Could you check a few things on this model? Use its own coordinates, in mm. A direction names the side the tool comes from. Give positions to 0.01 mm unless a question says otherwise; leave off trailing zeros. Loops run counter-clockwise (first coordinate to the right, second up) from the corner with the lowest first, then second, coordinate; pieces in that order, holes last. Notation, with made-up numbers: (-12.5, -39.5) - (5.5, -39.5) arc R20 ccw to (5.5, -35.5) - close; hole circle Ø10 at (9, 84). An arc over 180 degrees is marked (long way). One line per item, written item: value. Start each with the question number.
Q1. I want a section at B-B (y = -103.5). Please give me the cut outline in (x, z) (3 decimals).
Q2. I want a section at C-C (x = 100). Please give me the cut outline in (y, z) (3 decimals).
Q3. I'm going to push flat-ended pins straight in: P1, Ø6, axis at x = 45, z = 34.5, coming from the +Y side; P2, Ø18.5, axis at y = -9, z = 2, coming from the +X side; P3, Ø23, axis at x = 70.5, y = 7, coming from the -Z side (3 decimals). Where does each tip first touch, or does it pass through?
Q4. I want a section at A-A (z = 76.5). Please give me the cut outline in (x, y), then the cut area to 3 significant figures.
Q5. If I drill on line 1 (Z direction, x = 33.5, y = 68) (3 decimals); line 2 (Y direction, x = 41, z = 34.5); line 3 (X direction, y = -1.5, z = 75), over which ranges is the centre line in solid material (lowest first)? Write a range as from..to.
Q6. For faces 1 (the face through (88, 0, 15.875)), 2 (the face through (110.693, -9.728, 67.386)), 3 (the face through (33.269, 16.547, 50.986)), 4 (the face through (61, -2, 61.925)), 5 (the face through (23.73, -17, 18)), which set-ups out of +Z, -Z, +X, -X, +Y, -Y let a thin tool reach every point of the face, with its end or its side?
```python
from build123d import *

# Parameters (mm, degrees)
F1_DEPTH = 127
F0_W     = 25.4
F0_H     = 19.05
F2_DEPTH = 25.4
F3_DEPTH = 7.9375
F5_R     = 12.7


with BuildPart() as f1:
    # F0 (on Front) → F1 (new body, symmetric)
    with BuildSketch(Plane.XZ):
        Polygon((23.7298189036, 9.525), (-39.7701810964, 9.525), (-39.7701810964, -9.525), (42.7798189036, -9.525), (42.7798189036, 9.525), align=None)
    extrude(amount=F1_DEPTH, both=True)

    # F0 (on Front) → F2 (join, symmetric)
    with BuildSketch(Plane.XZ):
        with Locations((74.5298189036, 52.4002)):
            Rectangle(F0_W, F0_H)
        with BuildLine():
            Line((23.7298189036, 27.0002), (23.7298189036, 9.525))
            Line((23.7298189036, 9.525), (42.7798189036, 9.525))
            Line((42.7798189036, 9.525), (42.7798189036, 27.0002))
            ThreePointArc((42.7798189036, 27.0002), (47.4294987522, 38.2255201513), (58.6548189036, 42.8752))
            Line((58.6548189036, 42.8752), (61.8298189036, 42.8752))
            Line((61.8298189036, 42.8752), (61.8298189036, 61.9252))
            Line((61.8298189036, 61.9252), (58.6548189036, 61.9252))
            add(Edge.make_bspline(
                [(55.9463563883, 61.8200198703), (56.8425826502, 61.8608849379), (57.7453992228, 61.8959848389), (58.6548189036, 61.9252)],
                knots=[109.933459913, 109.933459913, 109.933459913, 109.933459913, 111.5045361635, 111.5045361635, 111.5045361635, 111.5045361635], degree=3))
            ThreePointArc((55.9463563883, 61.8200198703), (33.0194070837, 50.7189960451), (23.7298189036, 27.0002))
        make_face()
    extrude(amount=F2_DEPTH, both=True)

    # F0 (on Front) → F3 (join, symmetric)
    with BuildSketch(Plane.XZ):
        with BuildLine():
            add(Edge.make_bspline(
                [(-39.7701810964, 9.525), (-37.2096076888, 27.8732826741), (-6.7655926965, 58.9605544136), (55.9463563883, 61.8200198703)],
                knots=[0, 0, 0, 0, 109.933459913, 109.933459913, 109.933459913, 109.933459913], degree=3))
            Line((-39.7701810964, 9.525), (23.7298189036, 9.525))
            Line((23.7298189036, 9.525), (23.7298189036, 27.0002))
            ThreePointArc((23.7298189036, 27.0002), (33.0194070837, 50.7189960451), (55.9463563883, 61.8200198703))
        make_face()
    extrude(amount=F3_DEPTH, both=True)

    # F0 (on Front) → F4 (revolve)
    with BuildSketch(Plane.XZ):
        Polygon((87.2298189036, 117.475), (87.2298189036, 61.9252), (87.2298189036, 42.8752), (87.2298189036, 15.875), (112.6298189036, 15.875), (112.6298189036, 117.475), align=None)
    revolve(axis=Axis((87.2298189036, 0, 66.675), (0, 0, 1)))

    # F5
    f5_edges = [f1.edges().sort_by_distance(p)[0] for p in [
        (-39.770181, -127, 0),
        (42.779819, -127, 0),
        (42.779819, 127, 0),
        (-39.770181, 127, 0),
    ]]
    fillet(f5_edges, radius=F5_R)


solid = f1.part
```
Worked answers:
1. outline: (-39.77, -9.525) - (42.78, -9.525) - (42.78, 9.525) - (-39.77, 9.525) - close
2. outline: (-21.956, 15.875) - (21.956, 15.875) - (21.956, 117.475) - (-21.956, 117.475) - close
3. P1: stops at y = 25.4
3. P2: stops at x = 42.78
3. P3: stops at z = 15.875
4. outline: circle Ø50.8 at (87.23, 0)
4. area: 2,030 mm²
5. line 1: z = -9.525..9.525
5. line 2: y = -25.4..25.4
5. line 3: x = 61.87..112.59
6. face 1: -Z, +X, +Y, -Y
6. face 2: none
6. face 3: +Z, -X, +Y
6. face 4: +Z, -X
6. face 5: +Z, -X, -Y
